Answer from the drawing. Dimensions are ordinates in mm from the lowest x, y and z of the part. A direction names the side the tool comes from. Give positions to 0.01 mm unless a question says otherwise; leave off trailing zeros. Write each loop counter-clockwise with the first axis right and the second up, starting at its lowest first coordinate (ties: lowest second). Pieces come first, ordered by that corner, then holes. Notation, with made-up numbers: M 56,40 L 60,40 A28 ccw 60,72 Z; hole C 39,25.5 d3. An arc over 180 degrees is marked long. Put each result on its own line as item: value.
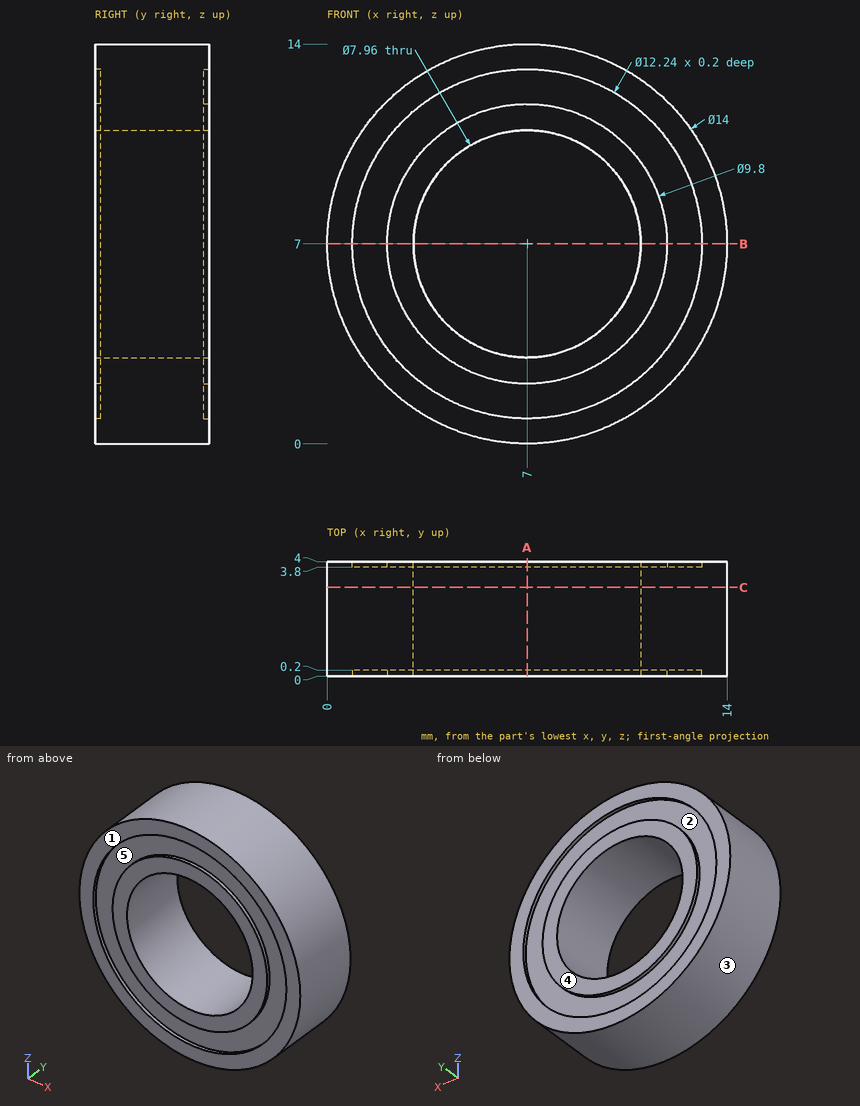
(1) For a pull along X with two mould halves and no side action, classify the marked faces 3, 4 and 5 as +X half, -X half, draft (parallel to the pull), parting line (faces both ways), or undercut.
Result:
face 3: parting line
face 4: draft
face 5: undercut
(2) Given pin 1 Ø2 at (y, z) = (1, 9.5) entering from +X; pin 2 Ø1 at (x, y) = (5, 3) entering from -Z; pin 3 Ø2 at (y, z) = (1, 3) entering from -X, each flat-ended and moving along its own axis, determine where each tip first touches the part or whether it passes through.
Result:
pin 1: stops at x = 13.84
pin 2: stops at z = 0.16
pin 3: stops at x = 0.68
(3) Which of the six approach directions +Z, -Z, +X, -X, +Y, -Y give full straight-line access (tool end or side, diameter ignored) to the marked faces 1 and 2?
Result:
face 1: +Z, -Z, +X, -X, -Y
face 2: +Y
(4) Section B-B on z = 7 is taken. Determine the outline of the cut face in (x, y).
Result:
outline: M 0,0 L 0.88,0 L 0.88,0.2 L 2.1,0.2 L 2.1,0 L 3.02,0 L 3.02,4 L 2.1,4 L 2.1,3.8 L 0.88,3.8 L 0.88,4 L 0,4 Z; M 10.98,0 L 11.9,0 L 11.9,0.2 L 13.12,0.2 L 13.12,0 L 14,0 L 14,4 L 13.12,4 L 13.12,3.8 L 11.9,3.8 L 11.9,4 L 10.98,4 Z
(5) Section C-C on y = 3.1 is taken. Determine the outline of the cut face in (x, z).
Result:
outline: C 7,7 d14; hole C 7,7 d7.96
(6) Straight lines are drawn through the part: line 1 along X through (y, z) = (3.9, 7); line 2 along Z through (x, y) = (7, 2.8). For each, find the intervals that lie inside material, in ascending order. Write a range as from..to.
Result:
line 1: x = 0..0.88, 2.1..3.02, 10.98..11.9, 13.12..14
line 2: z = 0..3.02, 10.98..14
(7) Section A-A on x = 7 is taken. Determine the outline of the cut face in (y, z), and give its area (3 significant figures).
Result:
outline: M 0,0 L 4,0 L 4,0.88 L 3.8,0.88 L 3.8,2.1 L 4,2.1 L 4,3.02 L 0,3.02 L 0,2.1 L 0.2,2.1 L 0.2,0.88 L 0,0.88 Z; M 0,10.98 L 4,10.98 L 4,11.9 L 3.8,11.9 L 3.8,13.12 L 4,13.12 L 4,14 L 0,14 L 0,13.12 L 0.2,13.12 L 0.2,11.9 L 0,11.9 Z
area: 23.2 mm²
